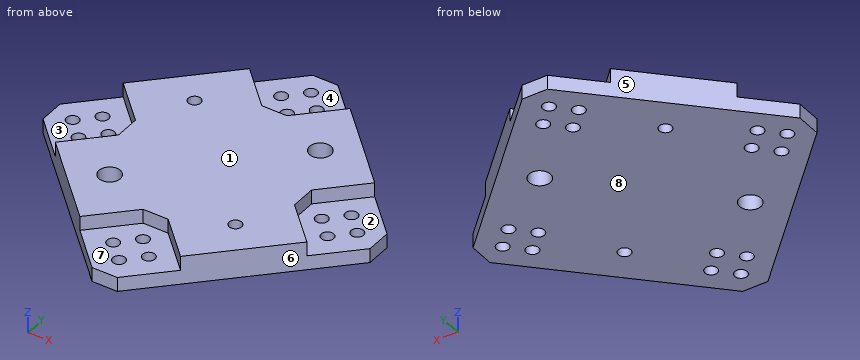
Autodesk Inventor part; units mm, degrees
ref_plane "YZ Plane" through (0, 0, 0) normal (1, 0, 0) x (0, 1, 0)
ref_plane "XZ Plane" through (0, 0, 0) normal (0, 1, 0) x (-1, 0, 0)
ref_plane "XY Plane" through (0, 0, 0) normal (0, 0, 1) x (1, 0, 0)
sketch "スケッチ2" plane through (0, 0, 0) normal (0, 0, 1) x (1, 0, 0)
  line L0 (0, -49.4975) -> (49.4975, 0)
  line L1 (49.4975, 0) -> (0, 49.4975)
  line L2 (0, 49.4975) -> (-49.4975, 0)
  line L3 (-49.4975, 0) -> (0, -49.4975)
  line L4 (0, -49.4975) -> (0, 49.4975) construction
  line L5 (49.4975, 0) -> (-49.4975, 0) construction
  circle A0 centre (-5, 35) radius 1.75
  circle A1 centre (5, 35) radius 1.75
  circle A2 centre (-35, -5) radius 1.75
  circle A3 centre (-35, 5) radius 1.75
  circle A4 centre (5, -35) radius 1.75
  circle A5 centre (-5, -35) radius 1.75
  circle A6 centre (35, 5) radius 1.75
  circle A7 centre (35, -5) radius 1.75
  line L6 (-24.7487, 24.7487) -> (24.7487, -24.7487) construction
  line L7 (24.7487, 24.7487) -> (-24.7487, -24.7487) construction
  circle A8 centre (17.6777, 17.6777) radius 3
  circle A9 centre (-17.6777, 17.6777) radius 1.75
  circle A10 centre (-17.6777, -17.6777) radius 3
  circle A11 centre (17.6777, -17.6777) radius 1.75
  circle A12 centre (-30, 0) radius 1.75
  circle A13 centre (-40, 0) radius 1.75
  line L8 (-35, -5) -> (-35, 5) construction
  circle A14 centre (0, -30) radius 1.75
  circle A15 centre (0, -40) radius 1.75
  circle A16 centre (30, 0) radius 1.75
  circle A17 centre (40, 0) radius 1.75
  circle A18 centre (0, 30) radius 1.75
  circle A19 centre (0, 40) radius 1.75
  point P0 (0, 0)
  dimension "d1" = 3.5
  dimension "d2" = 5
  dimension "d3" = 35
  dimension "d6" = 360
  dimension "d12" = 6
  dimension "d13" = 3.5
  dimension "d14" = 25
  dimension "d15" = 25
  dimension "d29" = 70
  dimension "d30" = 5
  dimension "d31" = 5
  dimension "d34" = 360
extrude "押し出し1" add sketch "スケッチ2" along normal blind 8
chamfer "面取り1" distance 5 angle 45 4 edges at (0, -49.4975, 4) (49.4975, 0, 4) (0, 49.4975, 4) (-49.4975, 0, 4)
sketch "スケッチ4" plane through (0, 0, 8) normal (0, 0, 1) x (1, 0, 0)
  line L0 (3.5355, -45.9619) -> (45.9619, -3.5355)
  line L1 (-45.9619, -3.5355) -> (-3.5355, -45.9619)
  line L2 (0, -21.2132) -> (14.1421, -35.3553)
  line L3 (14.1421, -35.3553) -> (0, -49.4975)
  line L4 (0, -49.4975) -> (-14.1421, -35.3553)
  line L5 (-14.1421, -35.3553) -> (0, -21.2132)
  line L6 (21.2132, 0) -> (35.3553, 14.1421)
  line L7 (35.3553, 14.1421) -> (49.4975, 0)
  line L8 (49.4975, 0) -> (35.3553, -14.1421)
  line L9 (35.3553, -14.1421) -> (21.2132, 0)
  line L10 (0, 21.2132) -> (-14.1421, 35.3553)
  line L11 (-14.1421, 35.3553) -> (0, 49.4975)
  line L12 (0, 49.4975) -> (14.1421, 35.3553)
  line L13 (14.1421, 35.3553) -> (0, 21.2132)
  line L14 (-21.2132, 0) -> (-35.3553, -14.1421)
  line L15 (-35.3553, -14.1421) -> (-49.4975, 0)
  line L16 (-49.4975, 0) -> (-35.3553, 14.1421)
  line L17 (-35.3553, 14.1421) -> (-21.2132, 0)
  point P0 (0, 0)
  point P1 (45.9619, 3.5355)
  point P2 (45.9619, -3.5355)
  point P3 (-3.5355, 45.9619)
  point P4 (3.5355, 45.9619)
  point P5 (-45.9619, -3.5355)
  point P6 (-45.9619, 3.5355)
  dimension "d36" = 20
  dimension "d37" = 20
  dimension "d40" = 360
extrude "押し出し3" cut sketch "スケッチ4" against normal blind 4
chamfer "面取り2" distance 5 angle 45 4 edges at (21.2132, 0, 6) (0, -21.2132, 6) (-21.2132, 0, 6) (0, 21.2132, 6)
properties part number "ワイヤジンバル1"
Work out the finished part from the listing and answer in its coordinate system (mm). Face numbers are marked on the shaded views. A direction names the side the tool comes from. Round coordinates to 2 decimals unless told otherwise and drop trailing zeros. Write each loop counter-clockwise with the first axis right and the second up, starting at its lowest first coordinate (ties: lowest second). Pieces come first, ordered by that corner, then holes.
1) A cutting plane is placed at C-C (z = 5.75). Give the vertices of the cut face in (x, y).
2) The mould has two halves that part along X. Classify the marked faces 5, 6, 7 and 8: pulls with the +X half, pulls with the -X half, needs draft (parallel to the pull), parting line crosses it, or undercut.
3) A cutting plane is placed at D-D (y = -40). Give the vertices of the cut face in (x, z).
4) A cutting plane is placed at A-A (y = 0). Give the vertices of the cut face in (x, z).
5) Given pin 1 Ø3 at (x, y) = (-40, 0) entering from -Z; pin 2 Ø5.5 at (x, y) = (0, 40) entering from +Z; pin 3 Ø2 at (x, z) = (35, 4) entering from +Y; pin 4 Ø2 at (y, z) = (-11, 6.5) entering from +X, each flat-ended and moving along its own axis, determine where each tip first touches the part or whether it passes through.
6) Straight lines are drawn through the part: line 1 (Y direction, x = 0, z = 2.2); line 2 (Y direction, x = 16.5, z = 3.25). For each, find the intervals that lie inside material, in ascending order.
7) A tool of negligible diameter and unlimited length cuts with its end or side. For the marked faces 1, 2, 3 and 4, from which of +Z, -Z, +X, -X, +Y, -Y can it reach the whole face along a straight path? Write none if from no direction.
Completed:
1. outline: (-35.36, -14.14) - (-14.14, -35.36) - (-3.54, -24.75) - (3.54, -24.75) - (14.14, -35.36) - (35.36, -14.14) - (24.75, -3.54) - (24.75, 3.54) - (35.36, 14.14) - (14.14, 35.36) - (3.54, 24.75) - (-3.54, 24.75) - (-14.14, 35.36) - (-35.36, 14.14) - (-24.75, 3.54) - (-24.75, -3.54) - close; hole circle Ø6 at (-17.68, -17.68); hole circle Ø3.5 at (-17.68, 17.68); hole circle Ø6 at (17.68, 17.68); hole circle Ø3.5 at (17.68, -17.68)
2. face 5: pulls with the -X half
2. face 6: pulls with the +X half
2. face 7: undercut
2. face 8: needs draft
3. outline: (-9.5, 0) - (-1.75, 0) - (-1.75, 4) - (-9.5, 4) - close; (1.75, 0) - (9.5, 0) - (9.5, 4) - (1.75, 4) - close
4. outline: (-45.96, 0) - (-41.75, 0) - (-41.75, 4) - (-45.96, 4) - close; (-38.25, 0) - (-31.75, 0) - (-31.75, 4) - (-38.25, 4) - close; (-28.25, 0) - (28.25, 0) - (28.25, 4) - (24.75, 4) - (24.75, 8) - (-24.75, 8) - (-24.75, 4) - (-28.25, 4) - close; (31.75, 0) - (38.25, 0) - (38.25, 4) - (31.75, 4) - close; (41.75, 0) - (45.96, 0) - (45.96, 4) - (41.75, 4) - close
5. pin 1: passes through
5. pin 2: stops at z = 4
5. pin 3: stops at y = 15.5
5. pin 4: stops at x = 33.21
6. line 1: y = -45.96 to -41.75, -38.25 to -31.75, -28.25 to 28.25, 31.75 to 38.25, 41.75 to 45.96
6. line 2: y = -33 to -18.97, -16.38 to 14.92, 20.44 to 33
7. face 1: +Z, +X, -X, +Y, -Y
7. face 2: +Z, +X
7. face 3: +Z, -X
7. face 4: +Z, +Y
